Could you check a few things on this drawing? It's one solid part, dimensions in mm from its lowest x, y, z. A direction names the side the tool comes from. Give positions to 0.01 mm unless a question says otherwise; leave off trailing zeros. Loops run counter-clockwise (first coordinate to the right, second up) from the corner with the lowest first, then second, coordinate; pieces in that order, holes last.
1. Imagine slicing it at C-C (y = 12). List the corners of the cut face in (x, z) for me.
2. For the marked faces 5 and 6, which set-ups out of +Z, -Z, +X, -X, +Y, -Y let a thin tool reach every point of the face, with its end or its side?
3. Imagine slicing it at B-B (x = 6.75). Count the separate pieces of the cut face and the enclosed holes in it.
4. Imagine slicing it at A-A (y = 6.5). List the corners of the cut face in (x, z) for me.
5. Thinking about a two-plate mould opening in X: for the marked faces 1, 2, 3 and 4, which applies, +X half, -X half, draft (parallel to the pull), parting line (faces both ways), or undercut?
6. For P1, Ø1.5, axis at x = 11.5, y = 8.5, coming from the -Z side; P2, Ø3, axis at x = 8, z = 7, coming from the -Y side, each with a flat end and sliding along its axis, tell me the tip position at first contact or that it passes through.
7. I need wall thicknesses on line 1 along X through (y, z) = (4.75, 7); line 2 along Z through (x, y) = (10, 2.75) (1 decimal); line 3 along Z through (x, y) = (4.25, 7.75). Which ranges of each line are inside material? Lowest first, please.
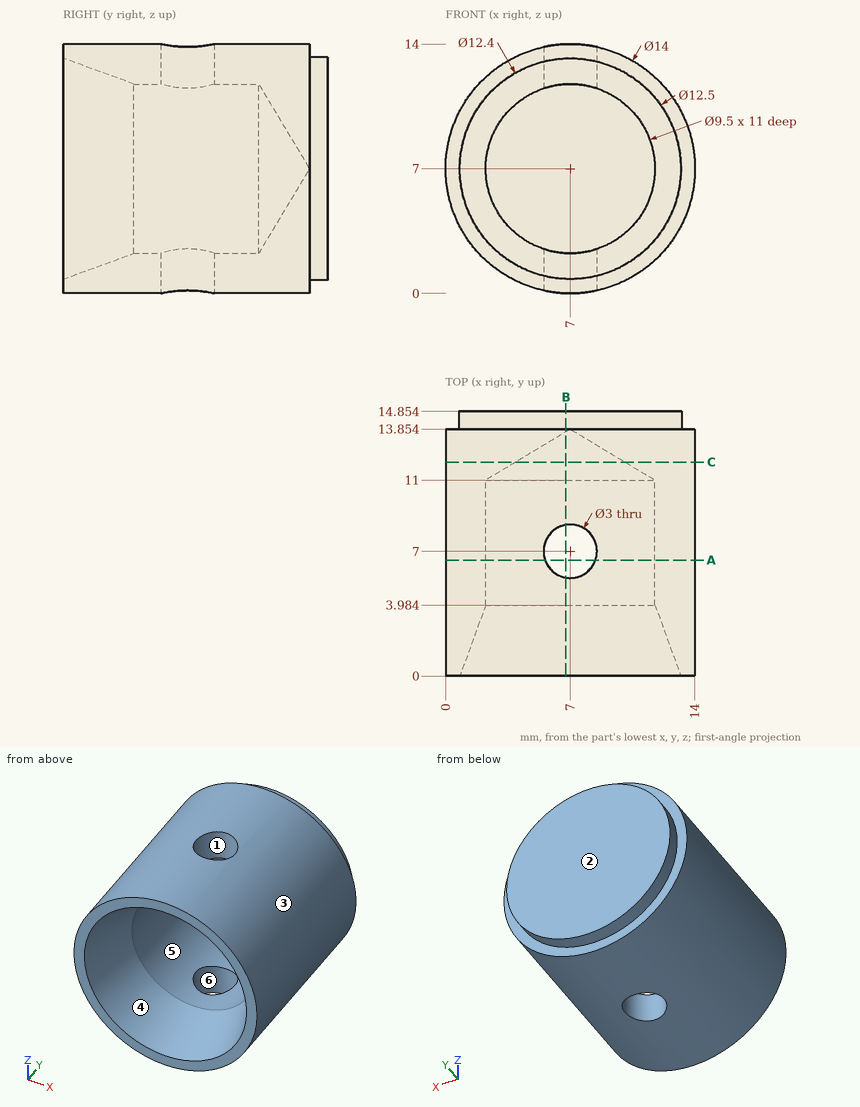
Derived:
1. outline: circle Ø14 at (7, 7); hole circle Ø6.17 at (7, 7)
2. face 5: -Y
2. face 6: +Z, -Z
3. separate pieces: 3
3. enclosed holes: 0
4. outline: (5.59, 0.14) - (5.59, 2.47) arc R4.75 cw to (5.59, 11.53) - (5.59, 13.86) arc R7 ccw to start; (8.41, 0.14) arc R7 ccw to (8.41, 13.86) - (8.41, 11.53) arc R4.75 cw to (8.41, 2.47) - close
5. face 1: undercut
5. face 2: draft
5. face 3: parting line
5. face 4: undercut
6. P1: stops at z = 1.09
6. P2: stops at y = 12.35
7. line 1: x = 0 to 2.25, 11.75 to 14
7. line 2: z = 0.7 to 2.8, 11.2 to 13.3
7. line 3: z = 0.56 to 3.13, 10.87 to 13.44
